Drawing for the job (mm, zero at the part's lowest x, y, z). A direction names the side the tool comes from. Coordinates: 2 decimals unless noted, no trailing zeros. Order: outer loops, then holes, each group sorted by start corner. A loop starts at its lowest first (then second) coordinate and runs counter-clockwise, first axis right, second up.
1) Wall check: L1, parallel to Y at x = 48.5, z = 6.5; L2, parallel to X at y = 37.7, z = 4; L3, parallel to Y at x = 50.5, z = 7.25 (1 decimal). Give the ranges that are in metal, low to high.
2) Tool access for the marked faces 1 and 2: list every direction of +Z, -Z, +X, -X, +Y, -Y with a clear straight run to the whole face (end or side of a thin tool).
3) Cut at A-A (z = 8). List the corners of the cut face in (x, y), and give its area (3 significant figures).
4) Cut at B-B (y = 19). List the corners of the cut face in (x, z).
5) Mould opens along Y. For the marked faces 3, 4 and 5 say: +Y half, -Y half, draft (parallel to the pull), parting line (faces both ways), or undercut.
6) Cut at D-D (z = 2.25). List the corners of the cut face in (x, y) (1 decimal), and give its area (3 significant figures).
7) Pin check, flat tips, straight feed: pin 1 Ø13.5 at (x, y) = (28, 22) entering from -Z; pin 2 Ø4.5 at (x, y) = (48.7, 6.7) entering from -Z. Stop position of each tip, or through.
8) Cut at C-C (y = 5.5). List the corners of the cut face in (x, z).
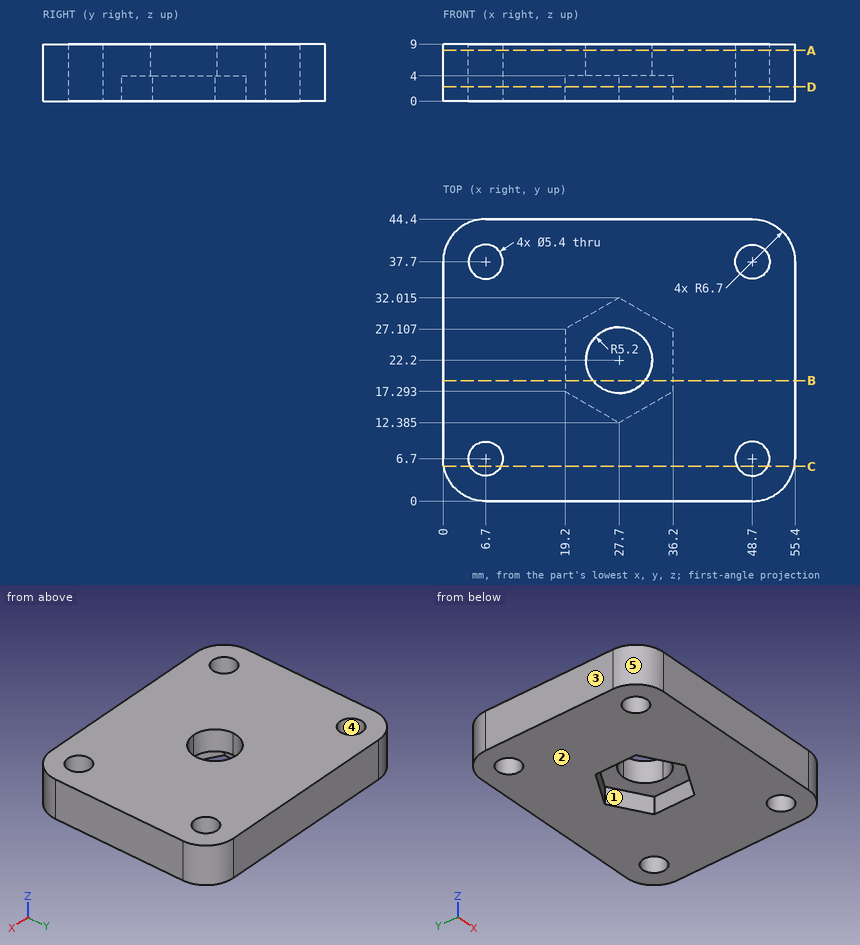
Geometry check:
1. L1: y = 0 to 4.01, 9.39 to 35.01, 40.39 to 44.4
1. L2: x = 0 to 4, 9.4 to 46, 51.4 to 55.4
1. L3: y = 0.2 to 4.7, 8.7 to 35.7, 39.7 to 44.2
2. face 1: -Z
2. face 2: -Z, +X, -X, +Y, -Y
3. outline: (0, 6.7) arc R6.7 ccw to (6.7, 0) - (48.7, 0) arc R6.7 ccw to (55.4, 6.7) - (55.4, 37.7) arc R6.7 ccw to (48.7, 44.4) - (6.7, 44.4) arc R6.7 ccw to (0, 37.7) - close; hole circle Ø5.4 at (6.7, 6.7); hole circle Ø5.4 at (6.7, 37.7); hole (22.5, 22.2) arc R5.2 ccw to (27.7, 17) arc R5.2 ccw to (32.9, 22.2) arc R5.2 ccw to (27.7, 27.4) arc R5.2 ccw to start; hole circle Ø5.4 at (48.7, 6.7); hole circle Ø5.4 at (48.7, 37.7)
3. area: 2,240 mm2
4. outline: (0, 0) - (19.2, 0) - (19.2, 4) - (23.6, 4) - (23.6, 9) - (0, 9) - close; (31.8, 4) - (36.2, 4) - (36.2, 0) - (55.4, 0) - (55.4, 9) - (31.8, 9) - close
5. face 3: draft
5. face 4: undercut
5. face 5: -Y half
6. outline: (0, 6.7) arc R6.7 ccw to (6.7, 0) - (48.7, 0) arc R6.7 ccw to (55.4, 6.7) - (55.4, 37.7) arc R6.7 ccw to (48.7, 44.4) - (6.7, 44.4) arc R6.7 ccw to (0, 37.7) - close; hole circle Ø5.4 at (6.7, 6.7); hole circle Ø5.4 at (6.7, 37.7); hole (19.2, 17.3) - (27.7, 12.4) - (36.2, 17.3) - (36.2, 27.1) - (27.7, 32) - (19.2, 27.1) - close; hole circle Ø5.4 at (48.7, 6.7); hole circle Ø5.4 at (48.7, 37.7)
6. area: 2,080 mm2
7. pin 1: stops at z = 4
7. pin 2: passes through
8. outline: (0.11, 0) - (4.28, 0) - (4.28, 9) - (0.11, 9) - close; (9.12, 0) - (46.28, 0) - (46.28, 9) - (9.12, 9) - close; (51.12, 0) - (55.29, 0) - (55.29, 9) - (51.12, 9) - close
